Verification items for the finished model (mm, model axes). Round coordinates to 2 decimals unless told otherwise and drop trailing zeros. Order: outer loops, then holes, each group sorted by start corner. A loop starts at its lowest first (then second) coordinate and runs counter-clockwise, first axis right, second up. Notation, with made-up numbers: (50, 14.25) -> (103, 14.25) arc R22 ccw to (103, 32.25) -> close; hole circle Ø9 at (-10, 62.5). An arc over 180 degrees is marked (long way). Answer in a Markdown table with one row per item. Add a question column.
Autodesk Inventor part; units mm, degrees
ref_plane "YZ Plane" through (0, 0, 0) normal (1, 0, 0) x (0, 1, 0)
ref_plane "XZ Plane" through (0, 0, 0) normal (0, 1, 0) x (-1, 0, 0)
ref_plane "XY Plane" through (0, 0, 0) normal (0, 0, 1) x (1, 0, 0)
sketch "Sketch1" plane through (0, 0, 0) normal (0, 1, 0) x (-1, 0, 0)
  line L0 (84.5044, -277.3965) -> (-445.7206, -277.3965)
  line L1 (-445.7206, -725.5287) -> (84.5044, -725.5287)
  line L2 (-445.7206, -277.3965) -> (-445.7206, -283.7465)
  line L3 (-445.7206, -283.7465) -> (-452.0706, -283.7465)
  line L4 (-452.0706, -302.7965) -> (-445.7206, -302.7965)
  line L5 (-445.7206, -302.7965) -> (-445.7206, -340.8965)
  line L6 (-445.7206, -340.8965) -> (-452.0706, -340.8965)
  line L7 (-452.0706, -359.9465) -> (-445.7206, -359.9465)
  line L8 (-445.7206, -359.9465) -> (-445.7206, -398.0465)
  line L9 (-445.7206, -398.0465) -> (-452.0706, -398.0465)
  line L10 (-452.0706, -417.0965) -> (-445.7206, -417.0965)
  line L11 (-445.7206, -417.0965) -> (-445.7206, -455.1965)
  line L12 (-445.7206, -455.1965) -> (-452.0706, -455.1965)
  line L13 (-452.0706, -474.2465) -> (-445.7206, -474.2465)
  line L14 (-445.7206, -512.3465) -> (-452.0706, -512.3465)
  line L15 (-452.0706, -531.3965) -> (-445.7206, -531.3965)
  line L16 (-445.7206, -531.3965) -> (-445.7206, -569.4965)
  line L17 (-445.7206, -569.4965) -> (-452.0706, -569.4965)
  line L18 (-452.0706, -588.5465) -> (-445.7206, -588.5465)
  line L19 (-445.7206, -588.5465) -> (-445.7206, -626.6465)
  line L20 (-445.7206, -626.6465) -> (-452.0706, -626.6465)
  line L21 (-452.0706, -645.6965) -> (-445.7206, -645.6965)
  line L22 (-445.7206, -645.6965) -> (-445.7206, -683.7965)
  line L23 (-445.7206, -683.7965) -> (-452.0706, -683.7965)
  line L24 (-452.0706, -702.8465) -> (-445.7206, -702.8465)
  line L25 (-445.7206, -702.8465) -> (-445.7206, -725.5287)
  line L26 (-452.0706, -283.7465) -> (-452.0706, -302.7965)
  line L27 (-452.0706, -340.8965) -> (-452.0706, -359.9465)
  line L28 (-452.0706, -398.0465) -> (-452.0706, -417.0965)
  line L29 (-452.0706, -455.1965) -> (-452.0706, -474.2465)
  line L30 (-452.0706, -512.3465) -> (-452.0706, -531.3965)
  line L31 (-452.0706, -569.4965) -> (-452.0706, -588.5465)
  line L32 (-452.0706, -626.6465) -> (-452.0706, -645.6965)
  line L33 (-452.0706, -683.7965) -> (-452.0706, -702.8465)
  line L34 (-445.7206, -512.3465) -> (-445.7206, -474.2465)
  line L35 (84.5044, -277.3965) -> (84.5044, -283.7465)
  line L36 (84.5044, -283.7465) -> (90.8544, -283.7465)
  line L37 (90.8544, -302.7965) -> (84.5044, -302.7965)
  line L38 (84.5044, -302.7965) -> (84.5044, -340.8965)
  line L39 (84.5044, -340.8965) -> (90.8544, -340.8965)
  line L40 (90.8544, -359.9465) -> (84.5044, -359.9465)
  line L41 (84.5044, -359.9465) -> (84.5044, -398.0465)
  line L42 (84.5044, -398.0465) -> (90.8544, -398.0465)
  line L43 (90.8544, -417.0965) -> (84.5044, -417.0965)
  line L44 (84.5044, -417.0965) -> (84.5044, -455.1965)
  line L45 (84.5044, -455.1965) -> (90.8544, -455.1965)
  line L46 (90.8544, -474.2465) -> (84.5044, -474.2465)
  line L47 (84.5044, -474.2465) -> (84.5044, -512.3465)
  line L48 (84.5044, -512.3465) -> (90.8544, -512.3465)
  line L49 (90.8544, -531.3965) -> (84.5044, -531.3965)
  line L50 (84.5044, -531.3965) -> (84.5044, -569.4965)
  line L51 (84.5044, -569.4965) -> (90.8544, -569.4965)
  line L52 (90.8544, -588.5465) -> (84.5044, -588.5465)
  line L53 (84.5044, -588.5465) -> (84.5044, -626.6465)
  line L54 (84.5044, -626.6465) -> (90.8544, -626.6465)
  line L55 (90.8544, -645.6965) -> (84.5044, -645.6965)
  line L56 (84.5044, -645.6965) -> (84.5044, -683.7965)
  line L57 (84.5044, -683.7965) -> (90.8544, -683.7965)
  line L58 (84.5044, -725.5287) -> (84.5044, -702.8465)
  line L59 (84.5044, -702.8465) -> (90.8544, -702.8465)
  line L60 (90.8544, -302.7965) -> (90.8544, -283.7465)
  line L61 (90.8544, -359.9465) -> (90.8544, -340.8965)
  line L62 (90.8544, -417.0965) -> (90.8544, -398.0465)
  line L63 (90.8544, -474.2465) -> (90.8544, -455.1965)
  line L64 (90.8544, -531.3965) -> (90.8544, -512.3465)
  line L65 (90.8544, -588.5465) -> (90.8544, -569.4965)
  line L66 (90.8544, -702.8465) -> (90.8544, -683.7965)
  line L67 (90.8544, -645.6965) -> (90.8544, -626.6465)
  line L68 (84.5044, -493.2965) -> (-445.7206, -493.2965)
  point P0 (0, 0)
  dimension "d53" = 6.35
  dimension "d54" = 38.1
  dimension "d55" = 19.05
  dimension "d56" = 19.05
  dimension "d57" = 19.05
  dimension "d58" = 38.1
  dimension "d59" = 38.1
  dimension "d60" = 19.05
  dimension "d61" = 38.1
  dimension "d62" = 19.05
  dimension "d63" = 38.1
  dimension "d64" = 19.05
  dimension "d65" = 38.1
  dimension "d66" = 19.05
  dimension "d67" = 38.1
  dimension "d68" = 19.05
  dimension "d69" = 6.35
  dimension "d70" = 6.35
  dimension "d71" = 6.35
  dimension "d72" = 6.35
  dimension "d74" = 6.35
  dimension "d75" = 6.35
  dimension "d76" = 6.35
  dimension "d94" = 22.6822
  dimension "d134" = 6.35
  dimension "d135" = 19.05
  dimension "d136" = 38.1
  dimension "d137" = 19.05
  dimension "d138" = 38.1
  dimension "d139" = 19.05
  dimension "d140" = 38.1
  dimension "d141" = 19.05
  dimension "d142" = 38.1
  dimension "d143" = 19.05
  dimension "d144" = 38.1
  dimension "d145" = 19.05
  dimension "d146" = 38.1
  dimension "d147" = 19.05
  dimension "d148" = 38.1
  dimension "d149" = 19.05
  dimension "d150" = 6.35
  dimension "d151" = 448.1322
  dimension "d152" = 542.925
extrude "Extrusion3" add sketch "Sketch1" along normal blind 6.35
properties part number "Back 2 V3"
1) Cross-section at A-A, the plane z = -673.5. Record the boundary of the cut face in (x, y).
2) Thickness scan on L1, parallel to X at y = 4.25, z = -682. Record the ranges inside material, lowest first. Write a range as [from, to].
3) Depth check by flat-ended pin: P1, Ø1.9, axis at x = 448, y = 3.5, coming from the +Z side; P2, Ø1.9, axis at y = 4, z = -718.5, coming from the -X side; P3, Ø1.9, axis at y = 3, z = -610, coming from the +X side. Enter the tip coordinate at first touch or a pass-through.
Results below:
| question | item | result |
|---|---|---|
| 1 | outline | (-84.5, 0) -> (445.72, 0) -> (445.72, 6.35) -> (-84.5, 6.35) -> close |
| 2 | L1 | [-84.5, 445.72] |
| 3 | P1 | z = -283.75 |
| 3 | P2 | x = -84.5 |
| 3 | P3 | x = 445.72 |
